```python
from build123d import *

# Parameters (mm, degrees)
SKETCH1_R           = 3.5
SKETCH1_R_2         = 2.05
BOSS_EXTRUDE1_DEPTH = 4
FILLET1_R           = 0.1


with BuildPart() as part:
    # Sketch1 → Boss-Extrude1 (new body)
    with BuildSketch(Plane(origin=(0, 0, 0), x_dir=(1, 0, 0), z_dir=(0, 1, 0))):
        with Locations(Location((0, 0, 0), (0, 0, 270))):
            Circle(SKETCH1_R)
        with Locations(Location((0, 0, 0), (0, 0, 270))):
            Circle(SKETCH1_R_2, mode=Mode.SUBTRACT)
    extrude(amount=BOSS_EXTRUDE1_DEPTH)

    # Fillet1
    fillet1_edges = [part.edges().sort_by_distance(p)[0] for p in [
        (0, 0, -3.5),
        (0, 4, -3.5),
        (0, 4, -2.05),
    ]]
    fillet(fillet1_edges, radius=FILLET1_R)


solid = part.part
```
The model under review builds one solid part; all positions refer to its coordinate system, in mm. Round coordinates to 2 decimals unless told otherwise and drop trailing zeros. Order: outer loops, then holes, each group sorted by start corner. A loop starts at its lowest first (then second) coordinate and runs counter-clockwise, first axis right, second up. Notation, with made-up numbers: (51, -3) -> (77, -3) arc R16 cw to (77, 25) -> close; hole circle Ø11 at (67.25, -28.5). An arc over 180 degrees is marked (long way). One line per item, written item: value. Start each with the question number.
Q1. Clearance check with flat-ended pins moving along their axes: pin 1 Ø1.5 at (x, y) = (-1, 3) entering from +Z; pin 2 Ø1 at (y, z) = (2.5, 2.5) entering from -X; pin 3 Ø1 at (y, z) = (1, 1) entering from +X. State where each tip first meets the part, or that it passes through.
Q2. Wall thickness on line 1 (X direction, y = 2.3, z = 0); line 2 (Z direction, x = -0.25, y = 1.4); line 3 (X direction, y = 1.5, z = -1.25): over which ranges is each line inside the solid? List them lowest first.
Q3. Take a section at B-B (z = 0). Write out the cut boundary in (x, y), and give its area (3 significant figures).
Q4. Take a section at C-C (y = 2.1). Write out the cut boundary in (x, z).
Q5. Take a section at A-A (x = 0). Write out the cut boundary in (y, z), and give its area (3 significant figures).
Reported:
1. pin 1: stops at z = 3.49
1. pin 2: stops at x = -2.87
1. pin 3: stops at x = 3.46
2. line 1: x = -3.5 to -2.05, 2.05 to 3.5
2. line 2: z = -3.49 to -2.03, 2.03 to 3.49
2. line 3: x = -3.27 to -1.62, 1.62 to 3.27
3. outline: (-3.5, 0.1) arc R0.1 ccw to (-3.4, 0) -> (-2.05, 0) -> (-2.05, 3.9) arc R0.1 ccw to (-2.15, 4) -> (-3.4, 4) arc R0.1 ccw to (-3.5, 3.9) -> close; (2.05, 0) -> (3.4, 0) arc R0.1 ccw to (3.5, 0.1) -> (3.5, 3.9) arc R0.1 ccw to (3.4, 4) -> (2.15, 4) arc R0.1 ccw to (2.05, 3.9) -> close
3. area: 11.6 mm2
4. outline: circle Ø7 at (0, 0); hole circle Ø4.1 at (0, 0)
5. outline: (0, -3.4) arc R0.1 ccw to (0.1, -3.5) -> (3.9, -3.5) arc R0.1 ccw to (4, -3.4) -> (4, -2.15) arc R0.1 ccw to (3.9, -2.05) -> (0, -2.05) -> close; (0, 2.05) -> (3.9, 2.05) arc R0.1 ccw to (4, 2.15) -> (4, 3.4) arc R0.1 ccw to (3.9, 3.5) -> (0.1, 3.5) arc R0.1 ccw to (0, 3.4) -> close
5. area: 11.6 mm2
